Check sheet for the drawn part. Datum: minimum x, y, z corner. Units: mm. A direction names the side the tool comes from. Round coordinates to 2 decimals unless told otherwise and drop trailing zeros. Write each loop counter-clockwise with the first axis right and the second up, starting at its lowest first coordinate (ties: lowest second). Pieces come first, ordered by that corner, then holes. Notation, with made-up numbers: (54.25, -33.75) - (104.25, -33.75) arc R19 ccw to (104.25, -23.75) - close; hole circle Ø3 at (65, 34). An arc over 180 degrees is marked (long way). Answer as a JSON object with one key per item and string values.
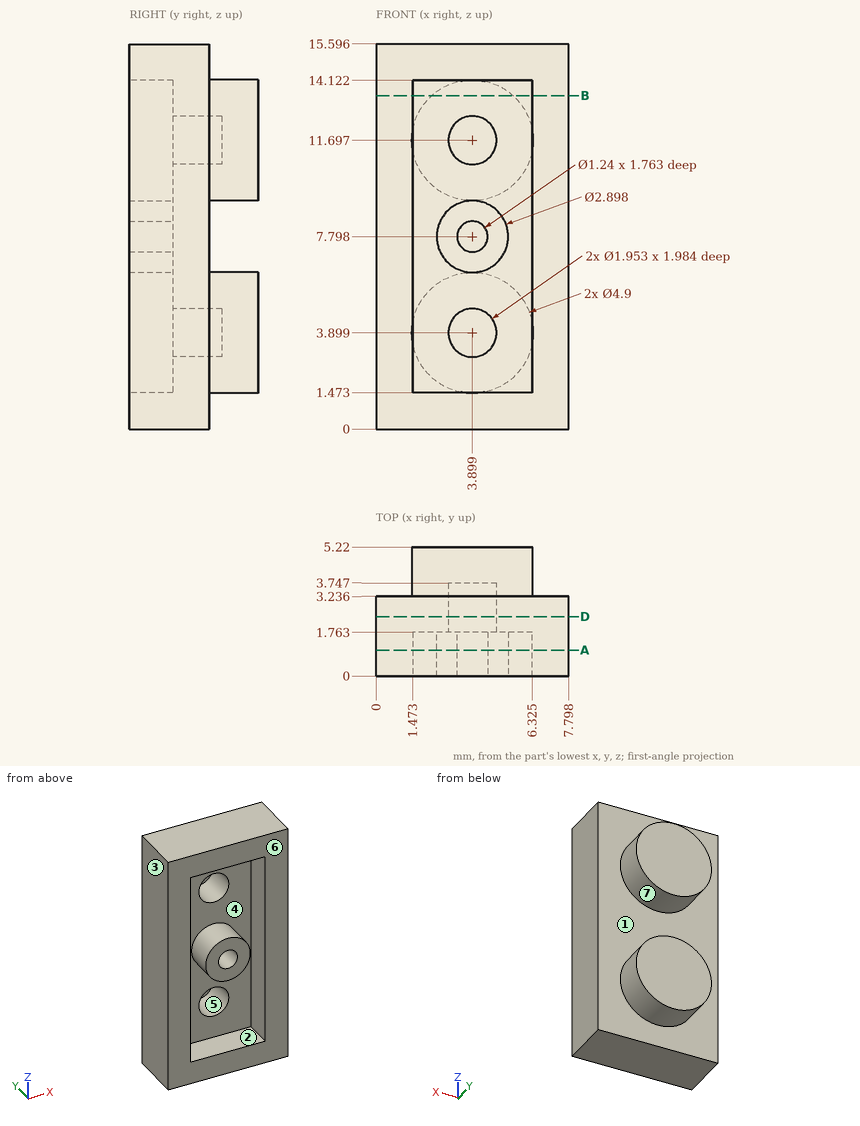
Q1. Release check for a two-part mould opening along X. For the marked faces 1, 2, 3 and 4 record: released by +X, released by -X, zero draft, split by the parting line, or undercut.
Geometry check:
{"face 1": "zero draft", "face 2": "undercut", "face 3": "released by -X", "face 4": "undercut"}
Q2. Material ranges on line 1 along X through (y, z) = (0.8, 5.75) (1 decimal); line 2 along Z through (x, y) = (6.25, 1.2) (1 decimal); line 3 along Y through (x, z) = (2.25, 5.25), recorded low to high. Write a range as [from, to].
Geometry check:
{"line 1": "x = [0, 1.5], [6.3, 7.8]", "line 2": "z = [0, 1.5], [14.1, 15.6]", "line 3": "y = [1.76, 5.22]"}
Q3. Set-up check for the marked faces 5, 6 and 7: record each of +Z, -Z, +X, -X, +Y, -Y from which the full face is reachable in a straight line by a thin tool's end or side.
Geometry check:
{"face 5": "-Y", "face 6": "+Z, -Z, +X, -X, -Y", "face 7": "+Y"}
Q4. Section check B-B, the plane z = 13.5. Record the cut outline in (x, y) (1 decimal).
Geometry check:
{"outline": "(0, 0) - (1.5, 0) - (1.5, 1.8) - (6.3, 1.8) - (6.3, 0) - (7.8, 0) - (7.8, 3.2) - (5.6, 3.2) - (5.6, 5.2) - (2.2, 5.2) - (2.2, 3.2) - (0, 3.2) - close"}
Q5. Section check D-D, the plane y = 2.4. Record the cut outline in (x, z) (1 decimal), then the cut area to 3 significant figures.
Geometry check:
{"outline": "(0, 0) - (7.8, 0) - (7.8, 15.6) - (0, 15.6) - close; hole circle Ø2 at (3.9, 3.9); hole circle Ø2 at (3.9, 11.7)", "area": "116 mm2"}
Q6. Gauge pin test, flat ends, axial feed: P1, Ø1.6, axis at x = 3.9, z = 3.9, coming from the -Y side; P2, Ø0.6, axis at x = 4, z = 8, coming from the -Y side. Record the tip position at first contact, or that the pin passes through.
Geometry check:
{"P1": "stops at y = 3.75", "P2": "stops at y = 1.76"}
Q7. Section check A-A, the plane y = 1.05. State how many separate pieces and enclosed holes the cut face has.
Geometry check:
{"separate pieces": "2", "enclosed holes": "2"}
